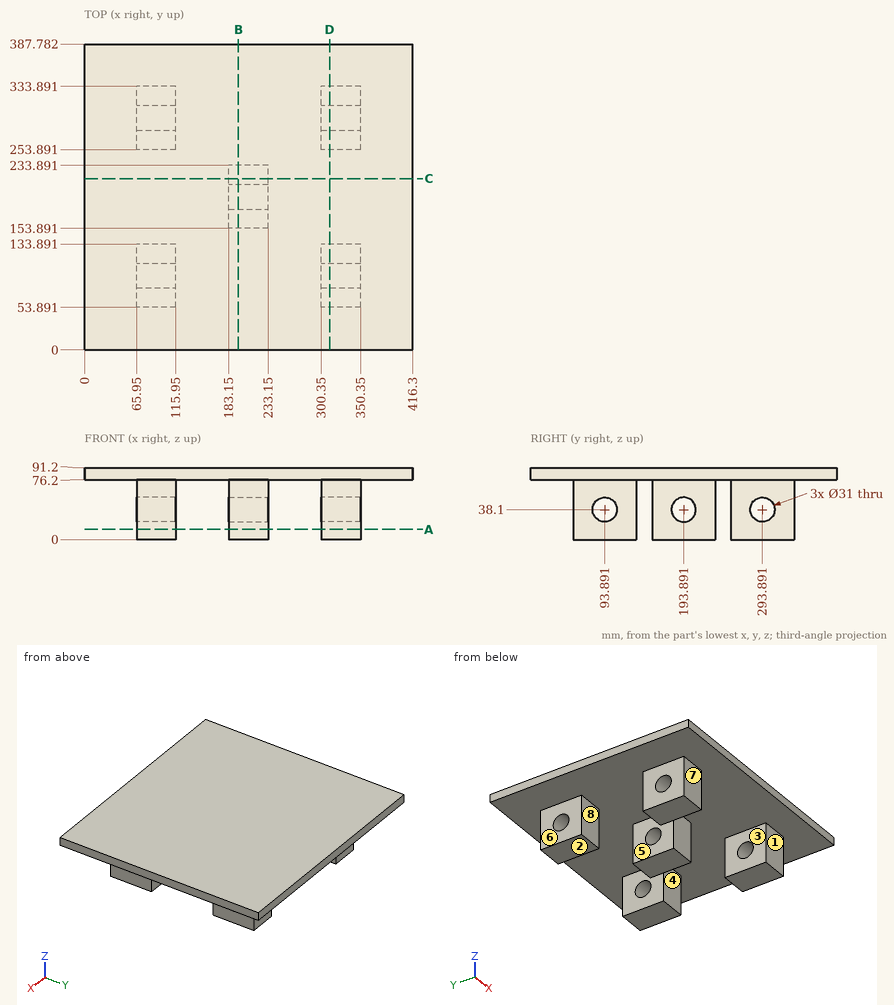
Verification items for this drawing (mm, ordinates from the low corner). A direction names the side the tool comes from. Coordinates: 2 decimals unless noted, no trailing zeros. Loops run counter-clockwise (first coordinate to the right, second up) from the corner with the lowest first, then second, coordinate; pieces in that order, holes last.
Item 1: Release check for a two-part mould opening along Y. For the marked faces 6, 7 and 8 record: released by +Y, released by -Y, zero draft, split by the parting line, or undercut.
Item 2: Sectioned sample at C-C, the plane y = 217. Record the boundary of the cut face in (x, z).
Item 3: Sectioned sample at A-A, the plane z = 13. Record the boundary of the cut face in (x, y), then the cut area to 3 significant figures.
Item 4: Go/stop test with flat-tipped pins: pin 1 Ø4 at (y, z) = (329, 25.5) entering from +X; pin 2 Ø15 at (x, z) = (316.5, 34.5) entering from +Y; pin 3 Ø15 at (x, z) = (206, 27) entering from -Y; pin 4 Ø5 at (x, y) = (89.5, 121) entering from -Z. Record where each tip stops, or that it passes through.
Item 5: Access from +Z, -Z, +X, -X, +Y, -Y to the whole of each face (thin tool, end or side, straight path). Record for the marked faces 1, 2, 3, 4 and 5.
Item 6: Sectioned sample at D-D, the plane x = 311. Record the boundary of the cut face in (y, z), then the cut area to 3 significant figures.
Item 7: Thickness scan on line 1 (Y direction, x = 81, z = 38); line 2 (X direction, y = 281.5, z = 13); line 3 (Y direction, x = 106.5, z = 50.5). Record the ranges inside material, lowest first.
Item 8: Sectioned sample at B-B, the plane x = 195. Record the boundary of the cut face in (y, z).
Check result:
1. face 6: zero draft
1. face 7: released by -Y
1. face 8: undercut
2. outline: (0, 76.2) - (183.15, 76.2) - (183.15, 0) - (233.15, 0) - (233.15, 76.2) - (416.3, 76.2) - (416.3, 91.2) - (0, 91.2) - close
3. outline: (65.95, 53.89) - (115.95, 53.89) - (115.95, 133.89) - (65.95, 133.89) - close; (65.95, 253.89) - (115.95, 253.89) - (115.95, 333.89) - (65.95, 333.89) - close; (183.15, 153.89) - (233.15, 153.89) - (233.15, 233.89) - (183.15, 233.89) - close; (300.35, 53.89) - (350.35, 53.89) - (350.35, 133.89) - (300.35, 133.89) - close; (300.35, 253.89) - (350.35, 253.89) - (350.35, 333.89) - (300.35, 333.89) - close
3. area: 20,000 mm2
4. pin 1: stops at x = 350.35
4. pin 2: stops at y = 333.89
4. pin 3: stops at y = 153.89
4. pin 4: stops at z = 0
5. face 1: -Z, +X, -X, -Y
5. face 2: -Z, +X, -X, +Y, -Y
5. face 3: -Z, +Y, -Y
5. face 4: -Z, +X, -X
5. face 5: -Z, -X, +Y, -Y
6. outline: (0, 76.2) - (53.89, 76.2) - (53.89, 0) - (133.89, 0) - (133.89, 76.2) - (253.89, 76.2) - (253.89, 0) - (333.89, 0) - (333.89, 76.2) - (387.78, 76.2) - (387.78, 91.2) - (0, 91.2) - close; hole circle Ø31 at (93.89, 38.1); hole circle Ø31 at (293.89, 38.1)
6. area: 16,500 mm2
7. line 1: y = 53.89 to 78.39, 109.39 to 133.89, 253.89 to 278.39, 309.39 to 333.89
7. line 2: x = 65.95 to 115.95, 300.35 to 350.35
7. line 3: y = 53.89 to 84.59, 103.19 to 133.89, 253.89 to 284.59, 303.19 to 333.89
8. outline: (0, 76.2) - (153.89, 76.2) - (153.89, 0) - (233.89, 0) - (233.89, 76.2) - (387.78, 76.2) - (387.78, 91.2) - (0, 91.2) - close; hole circle Ø31 at (193.89, 38.1)
